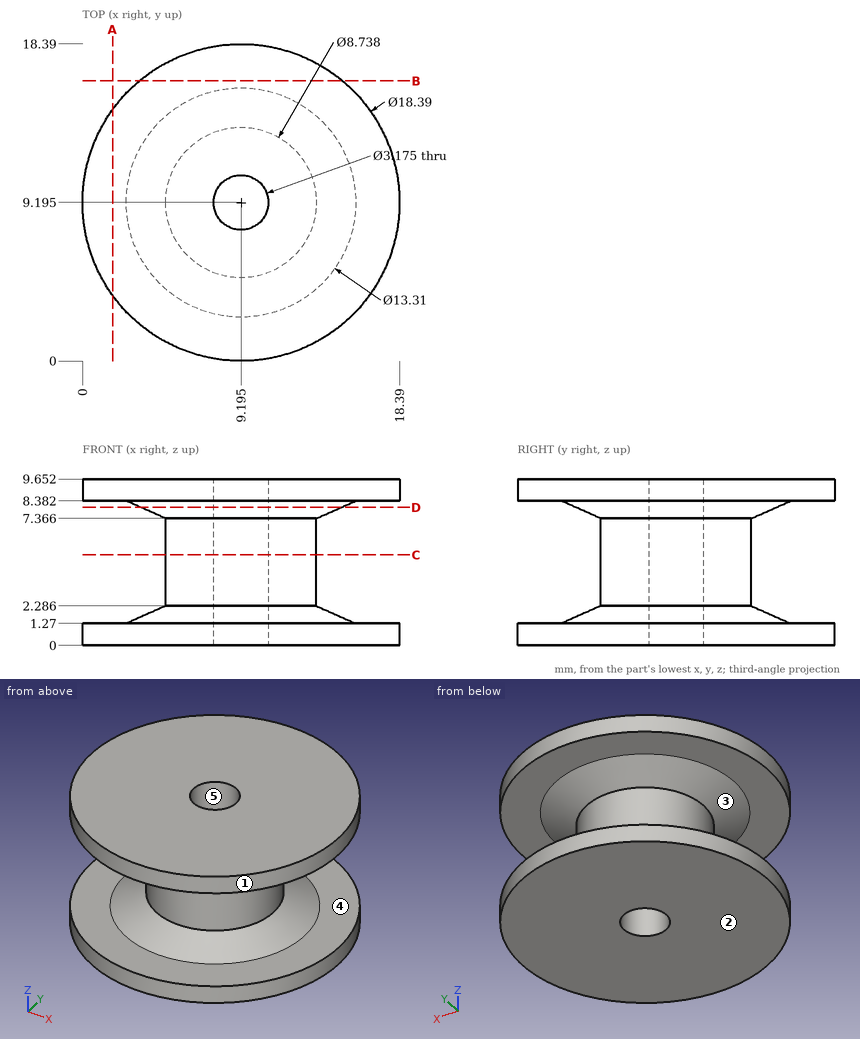
Geometry: see drawing. Coordinates: mm, zero at the bounding-box minimum. A direction names the side the tool comes from. Coordinates: 2 decimals unless noted, no trailing zeros. Order: outer loops, then holes, each group sorted by start corner. A loop starts at its lowest first (then second) coordinate and runs counter-clockwise, first axis right, second up. Notation, with made-up numbers: (-37.5, 20) - (-3.5, 20) arc R19 cw to (-3.5, 46) - close; hole circle Ø8 at (74, -2). An arc over 180 degrees is marked (long way). Write each question's results on one line, items separated by ' | '.
1) Pin query (flat end, axial travel): pin 1 (2 mm diameter, centred on x = 4.5, z = 3.5, fed in from +Y) (1 decimal); pin 2 (3 mm diameter, centred on y = 7.5, z = 1, fed in from -X); pin 3 (2 mm diameter, centred on y = 5.5, z = 6.5, fed in from +X); pin 4 (3 mm diameter, centred on x = 9.19, y = 9.19, fed in from +Z). Return the tip coordinate at first contact, or that it passes through.
Results list:
pin 1: y = 11.5 | pin 2: x = 0 | pin 3: x = 12.63 | pin 4: through
2) Set-up query: the marked faces 4 and 5. Return all of +Z, -Z, +X, -X, +Y, -Y with unobstructed straight access to the full face (end or side cutting, diameter ignored); none if empty.
Results list:
face 4: none | face 5: +Z, -Z
3) Pull-direction query (Z, two-part tool) for the marked faces 1, 2 and 3; classes: pulls with the +Z half, pulls with the -Z half, needs draft (parallel to the pull), parting line crosses it, or undercut.
Results list:
face 1: needs draft | face 2: pulls with the -Z half | face 3: undercut
4) Section C-C, the plane z = 5.25. Return loops of the section in (x, y) (1 decimal).
Results list:
outline: circle Ø8.7 at (9.2, 9.2); hole circle Ø3.2 at (9.2, 9.2)
5) Section B-B, the plane y = 16.25. Return loops of the section in (x, z).
Results list:
outline: (3.3, 0) - (15.09, 0) - (15.09, 1.27) - (3.3, 1.27) - close; (3.3, 8.38) - (15.09, 8.38) - (15.09, 9.65) - (3.3, 9.65) - close
6) Section D-D, the plane z = 8. Return loops of the section in (x, y) (1 decimal), plus the area to 3 significant figures.
Results list:
outline: circle Ø11.6 at (9.2, 9.2); hole circle Ø3.2 at (9.2, 9.2) | area: 97.6 mm^2
7) Line query: line 1 (Z direction, x = 2.75, y = 5.75); line 2 (X direction, y = 8.75, z = 6.75); line 3 (X direction, y = 9, z = 1.75) (1 decimal). Output: solid intervals per line, ascending. Write a range as from..to.
Results list:
line 1: 0..1.27, 8.38..9.65 | line 2: 4.85..7.67, 10.72..13.54 | line 3: 3.6..7.6, 10.8..14.8
8) Section A-A, the plane x = 1.75. Return loops of the section in (y, z).
Results list:
outline: (3.8, 0) - (14.59, 0) - (14.59, 1.27) - (3.8, 1.27) - close; (3.8, 8.38) - (14.59, 8.38) - (14.59, 9.65) - (3.8, 9.65) - close
